```python
from build123d import *

# Parameters (mm, degrees)
F0_R     = 35
F0_R_2   = 17.5
F1_DEPTH = 6
F3_DEPTH = 6.001


with BuildPart() as f1:
    # F0 (on Front) → F1 (new body)
    with BuildSketch(Plane.XZ):
        Circle(F0_R)
        Circle(F0_R_2, mode=Mode.SUBTRACT)
    extrude(amount=F1_DEPTH)

    # F2 (on face) → F3 (cut, through all)
    with BuildSketch(Plane.XZ.offset(6)):
        with BuildLine():
            ThreePointArc((16.454483, -9.5), (15.563889, -10.897952), (14.554844, -12.212965))
            Line((14.554844, -12.212965), (25.662489, -21.533385))
            ThreePointArc((25.662489, -21.533385), (27.441593, -19.214811), (29.011851, -16.75))
            Line((29.011851, -16.75), (16.454483, -9.5))
        make_face()
        with BuildLine():
            ThreePointArc((18.711347, -3.299315), (18.352591, -4.917562), (17.85416, -6.498383))
            Line((17.85416, -6.498383), (31.479703, -11.457675))
            ThreePointArc((31.479703, -11.457675), (32.358515, -8.670438), (32.99106, -5.817214))
            Line((32.99106, -5.817214), (18.711347, -3.299315))
        make_face()
        with BuildLine():
            ThreePointArc((18.711347, 3.299315), (18.927699, 1.655959), (19, 0))
            Line((19, 0), (33.5, 0))
            ThreePointArc((33.5, 0), (33.372522, 2.919717), (32.99106, 5.817214))
            Line((32.99106, 5.817214), (18.711347, 3.299315))
        make_face()
        with BuildLine():
            ThreePointArc((16.454483, 9.5), (17.219848, 8.029747), (17.85416, 6.498383))
            Line((17.85416, 6.498383), (31.479703, 11.457675))
            ThreePointArc((31.479703, 11.457675), (30.361311, 14.157712), (29.011851, 16.75))
            Line((29.011851, 16.75), (16.454483, 9.5))
        make_face()
        with BuildLine():
            ThreePointArc((6.498383, 17.85416), (8.029747, 17.219848), (9.5, 16.454483))
            Line((9.5, 16.454483), (16.75, 29.011851))
            ThreePointArc((16.75, 29.011851), (14.157712, 30.361311), (11.457675, 31.479703))
            Line((11.457675, 31.479703), (6.498383, 17.85416))
        make_face()
        with BuildLine():
            ThreePointArc((12.212965, 14.554844), (13.435029, 13.435029), (14.554844, 12.212965))
            Line((14.554844, 12.212965), (25.662489, 21.533385))
            ThreePointArc((25.662489, 21.533385), (23.688077, 23.688077), (21.533385, 25.662489))
            Line((21.533385, 25.662489), (12.212965, 14.554844))
        make_face()
        with BuildLine():
            ThreePointArc((0, 19), (1.655959, 18.927699), (3.299315, 18.711347))
            Line((3.299315, 18.711347), (5.817214, 32.99106))
            ThreePointArc((5.817214, 32.99106), (2.919717, 33.372522), (0, 33.5))
            Line((0, 33.5), (0, 19))
        make_face()
        with BuildLine():
            ThreePointArc((-6.498383, 17.85416), (-4.917562, 18.352591), (-3.299315, 18.711347))
            Line((-3.299315, 18.711347), (-5.817214, 32.99106))
            ThreePointArc((-5.817214, 32.99106), (-8.670438, 32.358515), (-11.457675, 31.479703))
            Line((-11.457675, 31.479703), (-6.498383, 17.85416))
        make_face()
        with BuildLine():
            ThreePointArc((-12.212965, 14.554844), (-10.897952, 15.563889), (-9.5, 16.454483))
            Line((-9.5, 16.454483), (-16.75, 29.011851))
            ThreePointArc((-16.75, 29.011851), (-19.214811, 27.441593), (-21.533385, 25.662489))
            Line((-21.533385, 25.662489), (-12.212965, 14.554844))
        make_face()
        with BuildLine():
            ThreePointArc((-16.454483, 9.5), (-15.563889, 10.897952), (-14.554844, 12.212965))
            Line((-14.554844, 12.212965), (-25.662489, 21.533385))
            ThreePointArc((-25.662489, 21.533385), (-27.441593, 19.214811), (-29.011851, 16.75))
            Line((-29.011851, 16.75), (-16.454483, 9.5))
        make_face()
        with BuildLine():
            ThreePointArc((-18.711347, 3.299315), (-18.352591, 4.917562), (-17.85416, 6.498383))
            Line((-17.85416, 6.498383), (-31.479703, 11.457675))
            ThreePointArc((-31.479703, 11.457675), (-32.358515, 8.670438), (-32.99106, 5.817214))
            Line((-32.99106, 5.817214), (-18.711347, 3.299315))
        make_face()
        with BuildLine():
            ThreePointArc((-12.212965, -14.554844), (-13.435029, -13.435029), (-14.554844, -12.212965))
            Line((-14.554844, -12.212965), (-25.662489, -21.533385))
            ThreePointArc((-25.662489, -21.533385), (-23.688077, -23.688077), (-21.533385, -25.662489))
            Line((-21.533385, -25.662489), (-12.212965, -14.554844))
        make_face()
        with BuildLine():
            ThreePointArc((-18.711347, -3.299315), (-18.927699, -1.655959), (-19, 0))
            Line((-19, 0), (-33.5, 0))
            ThreePointArc((-33.5, 0), (-33.372522, -2.919717), (-32.99106, -5.817214))
            Line((-32.99106, -5.817214), (-18.711347, -3.299315))
        make_face()
        with BuildLine():
            ThreePointArc((-16.454483, -9.5), (-17.219848, -8.029747), (-17.85416, -6.498383))
            Line((-17.85416, -6.498383), (-31.479703, -11.457675))
            ThreePointArc((-31.479703, -11.457675), (-30.361311, -14.157712), (-29.011851, -16.75))
            Line((-29.011851, -16.75), (-16.454483, -9.5))
        make_face()
        with BuildLine():
            ThreePointArc((0, -19), (-1.655959, -18.927699), (-3.299315, -18.711347))
            Line((-3.299315, -18.711347), (-5.817214, -32.99106))
            ThreePointArc((-5.817214, -32.99106), (-2.919717, -33.372522), (0, -33.5))
            Line((0, -33.5), (0, -19))
        make_face()
        with BuildLine():
            ThreePointArc((-6.498383, -17.85416), (-8.029747, -17.219848), (-9.5, -16.454483))
            Line((-9.5, -16.454483), (-16.75, -29.011851))
            ThreePointArc((-16.75, -29.011851), (-14.157712, -30.361311), (-11.457675, -31.479703))
            Line((-11.457675, -31.479703), (-6.498383, -17.85416))
        make_face()
        with BuildLine():
            ThreePointArc((6.498383, -17.85416), (4.917562, -18.352591), (3.299315, -18.711347))
            Line((3.299315, -18.711347), (5.817214, -32.99106))
            ThreePointArc((5.817214, -32.99106), (8.670438, -32.358515), (11.457675, -31.479703))
            Line((11.457675, -31.479703), (6.498383, -17.85416))
        make_face()
        with BuildLine():
            ThreePointArc((12.212965, -14.554844), (10.897952, -15.563889), (9.5, -16.454483))
            Line((9.5, -16.454483), (16.75, -29.011851))
            ThreePointArc((16.75, -29.011851), (19.214811, -27.441593), (21.533385, -25.662489))
            Line((21.533385, -25.662489), (12.212965, -14.554844))
        make_face()
    extrude(amount=-F3_DEPTH, mode=Mode.SUBTRACT)


solid = f1.part
```
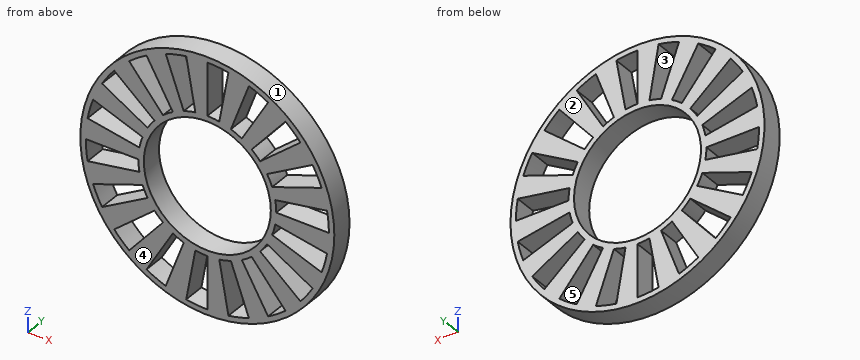
Work out the finished part from the listing and answer in its coordinate system (mm). Face numbers are marked on the shaded views. A direction names the side the tool comes from. Give positions to 0.01 mm unless a question says otherwise; leave off trailing zeros. Loops run counter-clockwise (first coordinate to the right, second up) from the corner with the lowest first, then second, coordinate; pieces in that order, holes last. Notation, with made-up numbers: (67, 29.5) -> (103, 29.5) arc R28 ccw to (103, 51.5) -> close; hole circle Ø7 at (42.5, 48.25). An arc over 180 degrees is marked (long way). One line per question, with ' | ' between items. Start each with the question number.
1) Determine the mould class of the marked faces 1, 2 and 3 for opening direction X: +X half, -X half, draft (parallel to the pull), parting line (faces both ways), or undercut.
2) For the marked faces 4 and 5, determine the directions among +Z, -Z, +X, -X, +Y, -Y from which every point of the face is accessible in a straight line to the end or side of a thin tool.
3) Section C-C, the plane x = -30 is taken. Determine the outline of the cut face in (y, z).
4) Each of these flat-tipped pins is pushed along its axis until it touches: pin 1 (2 mm diameter, centred on y = -1.5, z = 11.5, fed in from +X); pin 2 (5 mm diameter, centred on x = 20.5, z = -1, fed in from +Y); pin 3 (3 mm diameter, centred on y = -3, z = 26.5, fed in from +X); pin 4 (3 mm diameter, centred on x = -23.5, y = -4.5, fed in from -Z). Where does it stop, or does it pass through?
5) Section D-D, the plane y = -3.5 is taken. State how many separate pieces and enclosed holes the cut face has, then the cut area to 3 significant figures.
6) Section A-A, the plane x = 20 is taken. Determine the outline of the cut face in (y, z), then the cut area to 3 significant figures.
7) Section B-B, the plane z = 1 is taken. Determine the outline of the cut face in (x, y), then the cut area to 3 significant figures.
8) Straight lines are drawn through the part: L1, parallel to Z at x = 24, y = -4; L2, parallel to X at y = -1, z = 14; L3, parallel to X at y = -5, z = 1. For each, find the intervals that lie inside material, in ascending order.
Resolved:
1) face 1: parting line | face 2: draft | face 3: undercut
2) face 4: +Z, -Z, +X, -X, -Y | face 5: +Y, -Y
3) outline: (-6, -18.03) -> (0, -18.03) -> (0, -14.91) -> (-6, -14.91) -> close; (-6, -10.92) -> (0, -10.92) -> (0, -5.29) -> (-6, -5.29) -> close; (-6, 0) -> (0, 0) -> (0, 5.29) -> (-6, 5.29) -> close; (-6, 10.92) -> (0, 10.92) -> (0, 18.03) -> (-6, 18.03) -> close
4) pin 1: x = 33.39 | pin 2: y = 0 | pin 3: x = 24.49 | pin 4: z = -27.22
5) separate pieces: 1 | enclosed holes: 19 | area: 1,690 mm2
6) outline: (-6, -28.72) -> (0, -28.72) -> (0, -26.87) -> (-6, -26.87) -> close; (-6, -23.84) -> (0, -23.84) -> (0, -16.78) -> (-6, -16.78) -> close; (-6, -11.55) -> (0, -11.55) -> (0, -7.28) -> (-6, -7.28) -> close; (-6, -3.53) -> (0, -3.53) -> (0, 0) -> (-6, 0) -> close; (-6, 3.53) -> (0, 3.53) -> (0, 7.28) -> (-6, 7.28) -> close; (-6, 11.55) -> (0, 11.55) -> (0, 16.78) -> (-6, 16.78) -> close; (-6, 23.84) -> (0, 23.84) -> (0, 28.72) -> (-6, 28.72) -> close | area: 183 mm2
7) outline: (-34.99, -6) -> (-17.47, -6) -> (-17.47, 0) -> (-34.99, 0) -> close; (17.47, -6) -> (18.97, -6) -> (18.97, 0) -> (17.47, 0) -> close; (33.49, -6) -> (34.99, -6) -> (34.99, 0) -> (33.49, 0) -> close | area: 123 mm2
8) L1: -25.48 to -20.14, -13.86 to -8.74, -4.23 to 0, 4.23 to 8.74, 13.86 to 20.14, 23.37 to 25.48 | L2: -32.08 to -24.25, -16.68 to -10.5, 10.5 to 12.85, 16.68 to 24.25, 30.43 to 32.08 | L3: -34.99 to -17.47, 17.47 to 18.97, 33.49 to 34.99
